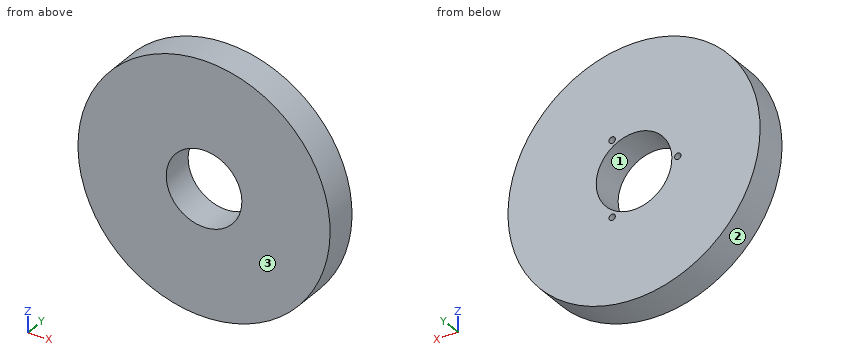
```python
from build123d import *

# Parameters (mm, degrees)
SKETCH1_R             = 75
BOSS_EXTRUDE1_DEPTH   = 20
SKETCH2_R             = 22.5
CUT_EXTRUDE1_DEPTH    = 108.935165725
SKETCH3_R             = 1.909197161
CUT_EXTRUDE2_DEPTH    = 18.190325
CIRPATTERN1_START     = 1.809675315
CIRPATTERN1_OUTLINE_R = 1.909197161
CIRPATTERN1_DEPTH     = 18.190324685


# Read off the part's stored shape, not the designer's step: CirPattern1
with BuildPart() as part:
    # Sketch1 → Boss-Extrude1 (new body)
    with BuildSketch(Plane(origin=(0, 0, 0), x_dir=(1, 0, 0), z_dir=(0, 1, 0))):
        with Locations(Location((0, 0, 0), (0, 0, 270))):
            Circle(SKETCH1_R)
    extrude(amount=BOSS_EXTRUDE1_DEPTH)

    # Sketch2 → Cut-Extrude1 (cut, through all)
    with BuildSketch(Plane(origin=(0, 0, 0), x_dir=(1, 0, 0), z_dir=(0, 1, 0))):
        with Locations(Location((0, 0, 0), (0, 0, 270))):
            Circle(SKETCH2_R)
    extrude(amount=CUT_EXTRUDE1_DEPTH, mode=Mode.SUBTRACT)

    # Sketch3 → Cut-Extrude2 (cut)
    with BuildSketch(Plane(origin=(0, 20, 0), x_dir=(1, 0, 0), z_dir=(0, 1, 0))):
        with Locations(Location((-26.053157287, 0, 0), (0, 0, 270))):
            Circle(SKETCH3_R)
    extrude(amount=-CUT_EXTRUDE2_DEPTH, mode=Mode.SUBTRACT)

    # CirPattern1 outline → CirPattern1 (cut)
    with BuildSketch(Plane(origin=(0, 0, 0), x_dir=(1, 0, 0), z_dir=(0, 1, 0)).offset(CIRPATTERN1_START)):
        with Locations((13.026578643, 22.562696059)):
            Circle(CIRPATTERN1_OUTLINE_R)
        with Locations((13.026578643, -22.562696059)):
            Circle(CIRPATTERN1_OUTLINE_R)
    extrude(amount=CIRPATTERN1_DEPTH, mode=Mode.SUBTRACT)


solid = part.part
```
Model file for the job. Use its own axes, mm. Face numbers are marked on the shaded views. Give positions to 0.01 mm unless a question says otherwise; leave off trailing zeros. Write each loop counter-clockwise with the first axis right and the second up, starting at its lowest first coordinate (ties: lowest second). Pieces come first, ordered by that corner, then holes. Notation, with made-up numbers: (62.5, 66) - (87.5, 66) arc R13 ccw to (87.5, 83) - close; hole circle Ø10 at (-33, 29.5). An arc over 180 degrees is marked (long way). One line per question, with ' | ' between items. Start each with the question number.
(1) Wall check: line 1 along X through (y, z) = (10.5, 0); line 2 along Z through (x, y) = (-16.5, 7.5); line 3 along Z through (x, y) = (-14, 5.75). Give the ranges that are in metal, low to high. Write a range as from..to.
(2) Pin check, flat tips, straight feed: P1, Ø2, axis at y = 18, z = 30, coming from the +X side; P2, Ø6, axis at y = 14, z = 9.5, coming from the +X side; P3, Ø1.1, axis at x = -26.5, z = -0.5, coming from the +Y side. Stop position of each tip, or through.
(3) Slice it at A-A on x = 0. Write the cut outline in (y, z), plus the area to 3 significant figures.
(4) Two-plate mould, pull along Z, no slides. Class the marked faces 1, 2 and 3: +Z half, -Z half, draft (parallel to the pull), parting line (faces both ways), or undercut.
(5) Slice it at B-B on z = 0. Write the cut outline in (x, y).
(6) Slice it at C-C on y = 5. Write the cut outline in (x, z).
(7) Slice it at D-D on z = -49.5. Write the cut outline in (x, y), plus the area to 3 significant figures.
Results below:
1) line 1: -75..-27.96, -24.14..-22.5, 22.5..75 | line 2: -73.16..-15.3, 15.3..73.16 | line 3: -73.68..-17.61, 17.61..73.68
2) P1: x = 69.17 | P2: x = 74.72 | P3: y = 1.81
3) outline: (0, -75) - (20, -75) - (20, -22.5) - (0, -22.5) - close; (0, 22.5) - (20, 22.5) - (20, 75) - (0, 75) - close | area: 2,100 mm^2
4) face 1: undercut | face 2: parting line | face 3: draft
5) outline: (-75, 0) - (-22.5, 0) - (-22.5, 20) - (-24.14, 20) - (-24.14, 1.81) - (-27.96, 1.81) - (-27.96, 20) - (-75, 20) - close; (22.5, 0) - (75, 0) - (75, 20) - (22.5, 20) - close
6) outline: circle Ø150 at (0, 0); hole circle Ø3.82 at (-26.05, 0); hole circle Ø45 at (0, 0); hole circle Ø3.82 at (13.03, -22.56); hole circle Ø3.82 at (13.03, 22.56)
7) outline: (-56.34, 0) - (56.34, 0) - (56.34, 20) - (-56.34, 20) - close | area: 2,250 mm^2
